Part model, mm, in its own coordinate system. A direction names the side the tool comes from. Coordinates: 2 decimals unless noted, no trailing zeros. Loops run counter-clockwise (first coordinate to the right, second up) from the corner with the lowest first, then second, coordinate; pieces in that order, holes last. Notation, with made-up numbers: (70, 80) - (120, 80) arc R21 ccw to (120, 118) - close; hole circle Ø10 at (48.5, 44). An arc over 180 degrees is marked (long way). Use a Markdown table: item, result. Add a question column.
1. 3-axis set-ups, long thin cutter, end or side, ignore diameter. For faces 1 (the flat face through (12, -3.175, -12)), 2 (the flat face through (5.5, -4.7, 3.2)): which of +Z, -Z, +X, -X, +Y, -Y reach the whole face in a straight line?
2. Band-saw the part on A-A, the plane x = 0. Give the cut face in (y, z) (3 decimals), plus the area to 3 significant figures.
3. Wall check: probe 1 along Z at (x, y) = (-11, -2.25); probe 2 along Y at (x, z) = (21, 3) (3 decimals); probe 3 along X at (y, z) = (-8.25, -2). Give the ranges that are in metal, low to high. Write a range as [from, to].
4. Band-saw the part on C-C, the plane x = -11. Count the separate pieces of the cut face and the enclosed holes in it, plus the area to 3 significant figures.
5. Pull direction Z, two halves, no side cores. Call faces 3 (the cylindrical face through (-10.57, -1.57, -18.52)), 4 (the flat face through (6, -9.525, 3)): pulls with the +Z half, pulls with the -Z half, needs draft (parallel to the pull), parting line crosses it, or undercut.
6. Band-saw the part on B-B, the plane y = -6.5. Give the cut face in (x, z), plus the area to 3 significant figures.
7. Drop flat-ended pins along their axis: pin 1 (6.5 mm diameter, centred on x = 11.91, z = -20.62, fed in from -Y) (3 decimals); pin 2 (2 mm diameter, centred on y = -2, z = 16, fed in from -X); pin 3 (3 mm diameter, centred on y = -7.5, z = -0.5, fed in from +X). Give the stop position or say it passes through.
from build123d import *

# Parameters (mm, degrees)
F0_R     = 28.575
F0_R_2   = 2.4892
F0_R_3   = 14.29512
F1_DEPTH = 3.175
F2_DEPTH = 9.525
F3_R     = 1.27


with BuildPart() as f1:
    # F0 (on Front) → F1 (new body)
    with BuildSketch(Plane.XZ):
        Circle(F0_R)
        with Locations((-11.90625, -20.62223)):
            Circle(F0_R_2, mode=Mode.SUBTRACT)
        with Locations((-20.62223, -11.90625)):
            Circle(F0_R_2, mode=Mode.SUBTRACT)
        with Locations((0, -23.8125)):
            Circle(F0_R_2, mode=Mode.SUBTRACT)
        with Locations((11.90625, -20.62223)):
            Circle(F0_R_2, mode=Mode.SUBTRACT)
        with Locations((20.62223, -11.90625)):
            Circle(F0_R_2, mode=Mode.SUBTRACT)
        with Locations((-23.8125, 0)):
            Circle(F0_R_2, mode=Mode.SUBTRACT)
        with Locations((-20.62223, 11.90625)):
            Circle(F0_R_2, mode=Mode.SUBTRACT)
        with Locations((-11.90625, 20.62223)):
            Circle(F0_R_2, mode=Mode.SUBTRACT)
        Circle(F0_R_3, mode=Mode.SUBTRACT)
        with Locations((23.8125, 0)):
            Circle(F0_R_2, mode=Mode.SUBTRACT)
        with Locations((20.62223, 11.90625)):
            Circle(F0_R_2, mode=Mode.SUBTRACT)
        with Locations((11.90625, 20.62223)):
            Circle(F0_R_2, mode=Mode.SUBTRACT)
        with Locations((0, 23.8125)):
            Circle(F0_R_2, mode=Mode.SUBTRACT)
        Circle(F0_R_3)
        Polygon((-7.347013, 0), (-3.673507, 6.3627), (3.673507, 6.3627), (7.347013, 0), (3.673507, -6.3627), (-3.673507, -6.3627), align=None, mode=Mode.SUBTRACT)
    extrude(amount=F1_DEPTH)

    # F0 (on Front) → F2 (join)
    with BuildSketch(Plane.XZ):
        Circle(F0_R_3)
        Polygon((-7.347013, 0), (-3.673507, 6.3627), (3.673507, 6.3627), (7.347013, 0), (3.673507, -6.3627), (-3.673507, -6.3627), align=None, mode=Mode.SUBTRACT)
    extrude(amount=F2_DEPTH)

    # F3
    f3_edges = [f1.edges().sort_by_distance(p)[0] for p in [
        (-28.575, -3.175, 0),
        (-14.29512, -9.525, 0),
        (-14.29512, -3.175, 0),
    ]]
    fillet(f3_edges, radius=F3_R)


solid = f1.part
Geometry check:
| question | item | result |
|---|---|---|
| 1 | face 1 | -Y |
| 1 | face 2 | +Y, -Y |
| 2 | outline | (-9.525, -13.025) arc R1.27 ccw to (-8.255, -14.295) - (-4.445, -14.295) arc R1.27 cw to (-3.175, -15.565) - (-3.175, -21.323) - (0, -21.323) - (0, -6.363) - (-9.525, -6.363) - close; (-9.525, 6.363) - (0, 6.363) - (0, 21.323) - (-3.175, 21.323) - (-3.175, 15.565) arc R1.27 cw to (-4.445, 14.295) - (-8.255, 14.295) arc R1.27 ccw to (-9.525, 13.025) - close; (-3.175, -27.305) arc R1.27 ccw to (-1.905, -28.575) - (0, -28.575) - (0, -26.302) - (-3.175, -26.302) - close; (-3.175, 26.302) - (0, 26.302) - (0, 28.575) - (-1.905, 28.575) arc R1.27 ccw to (-3.175, 27.305) - close |
| 2 | area | 209 mm^2 |
| 3 | probe 1 | z = [-26.32, -22.94], [-18.3, 18.3], [22.94, 26.32] |
| 3 | probe 2 | y = [-3.175, 0] |
| 3 | probe 3 | x = [-14.15, -6.19], [6.19, 14.15] |
| 4 | separate pieces | 3 |
| 4 | enclosed holes | 0 |
| 4 | area | 253 mm^2 |
| 5 | face 3 | undercut |
| 5 | face 4 | needs draft |
| 6 | outline | circle Ø28.59 at (0, 0); hole (-7.35, 0) - (-3.67, -6.36) - (3.67, -6.36) - (7.35, 0) - (3.67, 6.36) - (-3.67, 6.36) - close |
| 6 | area | 502 mm^2 |
| 7 | pin 1 | stops at y = -3.175 |
| 7 | pin 2 | stops at x = -24.32 |
| 7 | pin 3 | stops at x = 14.3 |
